Check sheet for the modelled part. Datum: model origin and axes. Units: mm. A direction names the side the tool comes from. Give positions to 0.01 mm unless a question says otherwise; leave off trailing zeros. Write each loop counter-clockwise with the first axis right and the second up, starting at its lowest first coordinate (ties: lowest second). Pieces come first, ordered by that corner, then holes. Notation, with made-up numbers: (64.25, 63.5) -> (69.25, 63.5) arc R19 ccw to (69.25, 98.5) -> close; hole circle Ø7 at (42, -26.75). An arc over 180 degrees is marked (long way). Use a Markdown table: item, result. Add a question column.
1. Cross-section at B-B (x = 38). Enter the section's corners in (y, z), then the cut area to 3 significant figures.
2. Cross-section at D-D (x = -32). Enter the section's corners in (y, z), then the cut area to 3 significant figures.
3. Cross-section at C-C (y = 11.5). Enter the section's corners in (x, z).
4. Scan lines: probe 1 along X at (y, z) = (-6, 0.8); probe 2 along Y at (x, z) = (33, 3.35); probe 3 along X at (y, z) = (-3, 1.05). Record each from-to range of solid material in increasing order. Write a range as [from, to].
5. Set-up check for faces 1 (the cylindrical face through (-35.299, 10.398, 2.535)), 2 (the flat face through (32, 6, 3.4)): record each of +Z, -Z, +X, -X, +Y, -Y from which the full face is reachable in a straight line by a thin tool's end or side.
6. Gauge pin test, flat ends, axial feed: P1, Ø2, axis at x = 32, y = 7.5, coming from the +Z side; P2, Ø2, axis at x = 32, y = 8, coming from the -Z side; P3, Ø3, axis at x = 28, z = 2, coming from the +Y side. Record the tip position at first contact, or that the pin passes through.
7. Cross-section at A-A (y = -7.5). Enter the section's corners in (x, z), then the cut area to 3 significant figures.
8. Release check for a two-part mould opening along X. For faces 3 (the cylindrical face through (-30.855, 7.86, 4.211)), 4 (the cylindrical face through (35.611, 10.225, 2.535)), 5 (the flat face through (23, 0, 0)) record: released by +X, released by -X, zero draft, split by the parting line, or undercut.
from build123d import *

# Parameters (mm, degrees)
SKETCH3_W           = 92
SKETCH3_H           = 31
BOSS_EXTRUDE2_DEPTH = 5
SKETCH4_R           = 103
SKETCH4_R_2         = 73
CUT_EXTRUDE1_DEPTH  = 6
SKETCH5_R           = 2.15
CUT_EXTRUDE2_DEPTH  = 6
CUT_EXTRUDE4_DEPTH  = 32
SKETCH8_R           = 1.2
CUT_EXTRUDE5_DEPTH  = 6
SKETCH9_R           = 2.1
CUT_EXTRUDE6_DEPTH  = 3.4


with BuildPart() as part:
    # Sketch3 → Boss-Extrude2 (new body)
    with BuildSketch(Plane.XY):
        Rectangle(SKETCH3_W, SKETCH3_H)
    extrude(amount=BOSS_EXTRUDE2_DEPTH)

    # Sketch4 → Cut-Extrude1 (cut, through all)
    with BuildSketch(Plane.XY.offset(5)):
        with Locations((0, -53.5)):
            Circle(SKETCH4_R)
        with Locations((0, -53.5)):
            Circle(SKETCH4_R_2, mode=Mode.SUBTRACT)
    extrude(amount=-CUT_EXTRUDE1_DEPTH, mode=Mode.SUBTRACT)

    # Sketch5 → Cut-Extrude2 (cut, through all)
    with BuildSketch(Plane.XY.offset(5)):
        with Locations((38, -7.5)):
            Circle(SKETCH5_R)
        with Locations((-38, -7.5)):
            Circle(SKETCH5_R)
    extrude(amount=-CUT_EXTRUDE2_DEPTH, mode=Mode.SUBTRACT)

    # Sketch7 → Cut-Extrude4 (cut, through all)
    with BuildSketch(Plane.XZ.offset(15.5)):
        Polygon((-1, 0), (0, 1.6), (1, 0), align=None)
    extrude(amount=-CUT_EXTRUDE4_DEPTH, mode=Mode.SUBTRACT)

    # Sketch8 → Cut-Extrude5 (cut, through all)
    with BuildSketch(Plane.XY.offset(5)):
        with Locations((-32, 7.5)):
            Circle(SKETCH8_R)
        with Locations((32, 7.5)):
            Circle(SKETCH8_R)
    extrude(amount=-CUT_EXTRUDE5_DEPTH, mode=Mode.SUBTRACT)

    # Sketch9 → Cut-Extrude6 (cut)
    with BuildSketch(Plane(origin=(0, 0, 0), x_dir=(-1, 0, 0), z_dir=(0, 0, -1))):
        with Locations((32, 7.5)):
            Circle(SKETCH9_R)
        with Locations((-32, 7.5)):
            Circle(SKETCH9_R)
    extrude(amount=-CUT_EXTRUDE6_DEPTH, mode=Mode.SUBTRACT)


solid = part.part
Worked answers:
| question | item | result |
|---|---|---|
| 1 | outline | (-15.5, 0) -> (-9.65, 0) -> (-9.65, 5) -> (-15.5, 5) -> close; (-5.35, 0) -> (8.83, 0) -> (8.83, 5) -> (-5.35, 5) -> close |
| 1 | area | 100 mm² |
| 2 | outline | (-15.5, 0) -> (5.4, 0) -> (5.4, 3.4) -> (6.3, 3.4) -> (6.3, 5) -> (-15.5, 5) -> close; (8.7, 3.4) -> (9.6, 3.4) -> (9.6, 0) -> (12.11, 0) -> (12.11, 5) -> (8.7, 5) -> close |
| 2 | area | 120 mm² |
| 3 | outline | (-33.23, 0) -> (-1, 0) -> (0, 1.6) -> (1, 0) -> (33.23, 0) -> (33.23, 5) -> (-33.23, 5) -> close |
| 4 | probe 1 | x = [-46, -39.54], [-36.46, -0.5], [0.5, 36.46], [39.54, 46] |
| 4 | probe 2 | y = [-15.5, 5.65], [9.35, 11.62] |
| 4 | probe 3 | x = [-46, -0.34], [0.34, 46] |
| 5 | face 1 | +Z, -Z, -X, +Y |
| 5 | face 2 | -Z |
| 6 | P1 | passes through |
| 6 | P2 | stops at z = 3.4 |
| 6 | P3 | stops at y = 14.52 |
| 7 | outline | (-46, 0) -> (-40.15, 0) -> (-40.15, 5) -> (-46, 5) -> close; (-35.85, 0) -> (-1, 0) -> (0, 1.6) -> (1, 0) -> (35.85, 0) -> (35.85, 5) -> (-35.85, 5) -> close; (40.15, 0) -> (46, 0) -> (46, 5) -> (40.15, 5) -> close |
| 7 | area | 415 mm² |
| 8 | face 3 | undercut |
| 8 | face 4 | released by +X |
| 8 | face 5 | zero draft |
